Input: dimensioned drawing with shaded views. Units: mm. Origin: part minimum x, y, z. Round coordinates to 2 decimals unless told otherwise and drop trailing zeros. Loops run counter-clockwise (first coordinate to the right, second up) from the corner with the lowest first, then second, coordinate; pieces in that order, holes last.
Item 1: Ray query, L1, parallel to Z at x = 32, y = 8.15; L2, parallel to X at y = 7.3, z = 53.6; L3, parallel to Z at x = 32, y = 3. Return the intervals inside material, ascending.
Item 2: Section query C-C on z = 63.2. Return loops of the section in (x, y) (1 decimal).
Item 3: First-contact query: P1, Ø4, axis at x = 63.75, z = 53.6, coming from the -Y side; P2, Ø9, axis at x = 8, z = 33.5, coming from the +Y side (3 decimals); P3, Ø9, axis at x = 63.75, z = 104.4, coming from the -Y side; P4, Ø5.5, axis at x = 5.5, z = 64.5, coming from the +Y side (3 decimals). Flat tips, straight axial feed; report the tip coordinate or a pass-through.
Item 4: Section query A-A on z = 104.4. Give the number of separate pieces and of enclosed holes in the cut face, then the cut area to 3 significant figures.
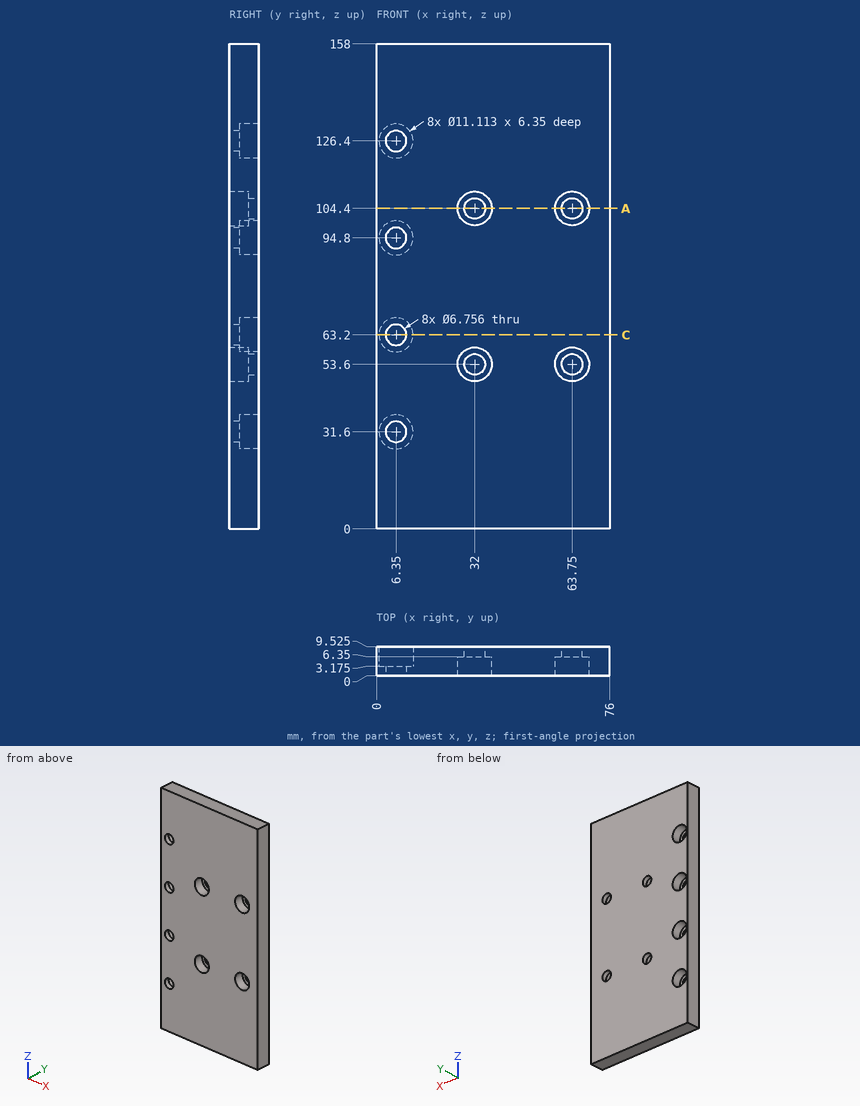
Data:
1. L1: z = 0 to 50.22, 56.98 to 101.02, 107.78 to 158
1. L2: x = 0 to 28.62, 35.38 to 60.37, 67.13 to 76
1. L3: z = 0 to 48.04, 59.16 to 98.84, 109.96 to 158
2. outline: (0, 0) - (3, 0) - (3, 3.2) - (0.8, 3.2) - (0.8, 9.5) - (0, 9.5) - close; (9.7, 0) - (76, 0) - (76, 9.5) - (11.9, 9.5) - (11.9, 3.2) - (9.7, 3.2) - close
3. P1: passes through
3. P2: stops at y = 9.525
3. P3: stops at y = 6.35
3. P4: stops at y = 3.175
4. separate pieces: 3
4. enclosed holes: 0
4. area: 540 mm2
